Design review of the part built by this model. Coordinates are the model's own, in mm. Face numbers are marked on the shaded views. Round coordinates to 2 decimals unless told otherwise and drop trailing zeros. Order: outer loops, then holes, each group sorted by start corner. A loop starts at its lowest first (then second) coordinate and runs counter-clockwise, first axis right, second up. Notation, with made-up numbers: (11.25, 57) - (25.25, 57) arc R14 cw to (25.25, 61) - close; hole circle Ø5 at (49, -24). An arc over 180 degrees is marked (long way). Use CSV: the item, a comma, the result in double quotes.
from build123d import *

# Parameters (mm, degrees)
BOSS_EXTRUDE1_DEPTH = 50
SKETCH3_R           = 2.5
CUT_EXTRUDE1_DEPTH  = 58.445626465


with BuildPart() as part:
    # Sketch2 → Boss-Extrude1 (new body)
    with BuildSketch(Plane.XY):
        with BuildLine():
            Line((-30, 26.457513111), (-30, -26.457513111))
            ThreePointArc((-30, -26.457513111), (-40, 0), (-30, 26.457513111))
        make_face()
    extrude(amount=BOSS_EXTRUDE1_DEPTH)

    # Sketch3 → Cut-Extrude1 (cut, through all)
    with BuildSketch(Plane(origin=(-30, 0, 0), x_dir=(0, 0, -1), z_dir=(1, 0, 0))):
        with Locations((-5, 0)):
            Circle(SKETCH3_R)
        with Locations((-15, -17.320508076)):
            Circle(SKETCH3_R)
        with Locations((-35, -17.320508076)):
            Circle(SKETCH3_R)
        with Locations((-45, 0)):
            Circle(SKETCH3_R)
        with Locations((-35, 17.320508076)):
            Circle(SKETCH3_R)
        with Locations((-15, 17.320508076)):
            Circle(SKETCH3_R)
    extrude(amount=-CUT_EXTRUDE1_DEPTH, mode=Mode.SUBTRACT)


solid = part.part
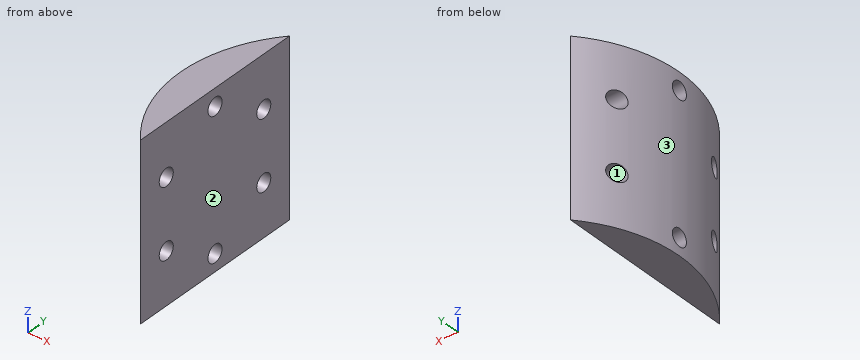
1) The part is to be moulded in two halves that separate along Y. For the marked faces 1, 2 and 3, say which applies: +Y half, -Y half, draft (parallel to the pull), parting line (faces both ways), or undercut.
Data:
face 1,"undercut"
face 2,"draft"
face 3,"parting line"
2) We need section C-C (x = -30.75). Give the boundary of the cut face in (y, z), then the cut area to 3 significant figures.
Data:
outline,"(-25.58, 0) - (25.58, 0) - (25.58, 50) - (-25.58, 50) - close; hole circle Ø5 at (-17.32, 15); hole circle Ø5 at (-17.32, 35); hole circle Ø5 at (0, 5); hole circle Ø5 at (0, 45); hole circle Ø5 at (17.32, 15); hole circle Ø5 at (17.32, 35)"
area,"2,440 mm2"
3) Insertion check: pin 1 Ø6 at (x, y) = (-38.5, 12.5) entering from +Z; pin 2 Ø2 at (x, z) = (-36, 17.5) entering from +Y; pin 3 Ø6 at (y, z) = (-17.32, 15) entering from -X. Each pin has a flat end and moves straight along its axis. Give the tip position at first contact, or say it passes through.
Data:
pin 1,"stops at z = 50"
pin 2,"stops at y = 19.36"
pin 3,"stops at x = -37.35"
4) We need section D-D (z = 5.5). Give the boundary of the cut face in (x, y).
Data:
outline,"(-39.92, -2.45) arc R40 ccw to (-30, -26.46) - (-30, -2.45) - close; (-39.92, 2.45) - (-30, 2.45) - (-30, 26.46) arc R40 ccw to start"
5) To check wall thickness, follow L1, parallel to Z at x = -39, y = 0; L2, parallel to Y at x = -33, z = 35; L3, parallel to Z at x = -34, y = -1.5. State the ranges of each line that lie inside material, in increasing order. Write a range as from..to.
Data:
L1,"z = 0..2.5, 7.5..42.5, 47.5..50"
L2,"y = -22.61..-19.82, -14.82..14.82, 19.82..22.61"
L3,"z = 0..3, 7..43, 47..50"
6) We need section A-A (y = 0). Give the boundary of the cut face in (x, z), then the cut area to 3 significant figures.
Data:
outline,"(-40, 0) - (-30, 0) - (-30, 2.5) - (-40, 2.5) - close; (-40, 7.5) - (-30, 7.5) - (-30, 42.5) - (-40, 42.5) - close; (-40, 47.5) - (-30, 47.5) - (-30, 50) - (-40, 50) - close"
area,"400 mm2"
7) We need section B-B (z = 15). Give the boundary of the cut face in (x, y), then the cut area to 3 significant figures.
Data:
outline,"(-37.15, -14.82) - (-30, -14.82) - (-30, 14.82) - (-37.15, 14.82) arc R40 ccw to start; (-34.74, -19.82) arc R40 ccw to (-30, -26.46) - (-30, -19.82) - close; (-34.74, 19.82) - (-30, 19.82) - (-30, 26.46) arc R40 ccw to start"
area,"302 mm2"
